from build123d import *

# Parameters (mm, degrees)
SKETCH1_W           = 63.5
SKETCH1_H           = 12.7
BOSS_EXTRUDE1_DEPTH = 1.27
FILLET1_R           = 2.54


with BuildPart() as part:
    # Sketch1 → Boss-Extrude1 (new body)
    with BuildSketch(Plane(origin=(0, 0, 0), x_dir=(1, 0, 0), z_dir=(0, 1, 0))):
        Rectangle(SKETCH1_W, SKETCH1_H)
        with BuildLine():
            Line((25.4, 2.286), (27.94, 2.286))
            ThreePointArc((27.94, 2.286), (30.226, 0), (27.94, -2.286))
            Line((27.94, -2.286), (25.4, -2.286))
            ThreePointArc((25.4, -2.286), (23.114, 0), (25.4, 2.286))
        make_face(mode=Mode.SUBTRACT)
        with BuildLine():
            Line((-27.94, 2.286), (-25.4, 2.286))
            ThreePointArc((-25.4, 2.286), (-23.114, 0), (-25.4, -2.286))
            Line((-25.4, -2.286), (-27.94, -2.286))
            ThreePointArc((-27.94, -2.286), (-30.226, 0), (-27.94, 2.286))
        make_face(mode=Mode.SUBTRACT)
    extrude(amount=BOSS_EXTRUDE1_DEPTH)

    # Fillet1
    fillet1_edges = [part.edges().sort_by_distance(p)[0] for p in [
        (-31.75, 0.635, -6.35),
        (31.75, 0.635, -6.35),
        (31.75, 0.635, 6.35),
        (-31.75, 0.635, 6.35),
    ]]
    fillet(fillet1_edges, radius=FILLET1_R)


solid = part.part
The listing builds one solid part. Answer for the finished solid, in the listing's coordinates (mm). A direction names the side the tool comes from. Coordinates: 2 decimals unless noted, no trailing zeros. Loops run counter-clockwise (first coordinate to the right, second up) from the corner with the lowest first, then second, coordinate; pieces in that order, holes last.
1) A flat-ended cylindrical pin translates along its axis: pin 1 Ø3 at (x, z) = (1.5, 1) entering from -Y. Find the tip coordinate at first contact, or state that the pin passes through.
2) Determine the mould class of faces 1 (the face through (27, 1, 2.286)), 2 (the face through (-31.026, 0.644, -5.586)), 3 (the face through (31.75, 1, 0)) for opening direction X: pulls with the +X half, pulls with the -X half, needs draft (parallel to the pull), parting line crosses it, or undercut.
3) Find section C-C on x = -24. Write down the section's boundary in (y, z), then the cut area to 3 significant figures.
4) A tool of negligible diameter and unlimited length cuts with its end or side. For faces 4 (the face through (0, 0, 0)), 5 (the face through (30.225, 0.626, -0.05)), from which of +Z, -Z, +X, -X, +Y, -Y can it reach the whole face along a straight path? Write none if from no direction.
5) Find section B-B on z = 0. Write down the section's boundary in (x, y).
6) Find section A-A on y = 0.45. Write down the section's boundary in (x, z).
7) Find the intervals of material crossed by L1, parallel to X at y = 0.6, z = -0.25; L2, parallel to X at y = 0.55, z = 1; L3, parallel to X at y = 0.85, z = -4, in increasing order.
Values:
1. pin 1: stops at y = 0
2. face 1: undercut
2. face 2: pulls with the -X half
2. face 3: pulls with the +X half
3. outline: (0, -6.35) - (1.27, -6.35) - (1.27, -1.81) - (0, -1.81) - close; (0, 1.81) - (1.27, 1.81) - (1.27, 6.35) - (0, 6.35) - close
3. area: 11.5 mm2
4. face 4: +Z, -Z, +X, -X, -Y
4. face 5: +Y, -Y
5. outline: (-31.75, 0) - (-30.23, 0) - (-30.23, 1.27) - (-31.75, 1.27) - close; (-23.11, 0) - (23.11, 0) - (23.11, 1.27) - (-23.11, 1.27) - close; (30.23, 0) - (31.75, 0) - (31.75, 1.27) - (30.23, 1.27) - close
6. outline: (-31.75, -3.81) arc R2.54 ccw to (-29.21, -6.35) - (29.21, -6.35) arc R2.54 ccw to (31.75, -3.81) - (31.75, 3.81) arc R2.54 ccw to (29.21, 6.35) - (-29.21, 6.35) arc R2.54 ccw to (-31.75, 3.81) - close; hole (-27.94, -2.29) - (-25.4, -2.29) arc R2.29 ccw to (-25.4, 2.29) - (-27.94, 2.29) arc R2.29 ccw to start; hole (25.4, -2.29) - (27.94, -2.29) arc R2.29 ccw to (27.94, 2.29) - (25.4, 2.29) arc R2.29 ccw to start
7. L1: x = -31.75 to -30.21, -23.13 to 23.13, 30.21 to 31.75
7. L2: x = -31.75 to -30, -23.34 to 23.34, 30 to 31.75
7. L3: x = -31.74 to 31.74
